The model under review builds one solid part; all positions refer to its coordinate system, in mm. Coordinates: 2 decimals unless noted, no trailing zeros. Write each loop counter-clockwise with the first axis right and the second up, starting at its lowest first coordinate (ties: lowest second). Pieces come first, ordered by that corner, then holes. Notation, with made-up numbers: (-15, -20) -> (0, -20) arc R8 ccw to (0, -8) -> close; hole circle Ø2 at (84.5, 24.25). An arc over 180 degrees is marked (long way). Put each result on its own line as item: value. Start each with the question number.
from build123d import *

# Parameters (mm, degrees)
F1_DEPTH = 10


with BuildPart() as f1:
    # F0 (on Top) → F1 (new body)
    with BuildSketch(Plane.XY):
        with BuildLine():
            Line((3.8890872965, 3.8890872965), (3.1819805153, 3.1819805153))
            ThreePointArc((3.1819805153, 3.1819805153), (4.1574578963, 1.7220754456), (4.5, 0))
            ThreePointArc((4.5, 0), (3.1819805153, -3.1819805153), (0, -4.5))
            Line((0, -4.5), (0, -5.5))
            ThreePointArc((0, -5.5), (3.8890872965, -3.8890872965), (5.5, 0))
            ThreePointArc((5.5, 0), (5.0813374288, 2.104758878), (3.8890872965, 3.8890872965))
        make_face()
        with BuildLine():
            Line((4.5961940777, 4.5961940777), (3.8890872965, 3.8890872965))
            ThreePointArc((3.8890872965, 3.8890872965), (5.0813374288, 2.104758878), (5.5, 0))
            ThreePointArc((5.5, 0), (3.8890872965, -3.8890872965), (0, -5.5))
            Line((0, -5.5), (0, -6.5))
            ThreePointArc((0, -6.5), (4.5961940777, -4.5961940777), (6.5, 0))
            ThreePointArc((6.5, 0), (6.0052169613, 2.4874423104), (4.5961940777, 4.5961940777))
        make_face()
        with BuildLine():
            Line((5.6568542495, 5.6568542495), (4.5961940777, 4.5961940777))
            ThreePointArc((4.5961940777, 4.5961940777), (6.0052169613, 2.4874423104), (6.5, 0))
            ThreePointArc((6.5, 0), (4.5961940777, -4.5961940777), (0, -6.5))
            Line((0, -6.5), (0, -8))
            ThreePointArc((0, -8), (5.6568542495, -5.6568542495), (8, 0))
            ThreePointArc((8, 0), (7.3910362601, 3.0614674589), (5.6568542495, 5.6568542495))
        make_face()
        with BuildLine():
            Line((6.3639610307, 6.3639610307), (5.6568542495, 5.6568542495))
            ThreePointArc((5.6568542495, 5.6568542495), (7.3910362601, 3.0614674589), (8, 0))
            ThreePointArc((8, 0), (5.6568542495, -5.6568542495), (0, -8))
            Line((0, -8), (0, -9))
            ThreePointArc((0, -9), (6.3639610307, -6.3639610307), (9, 0))
            ThreePointArc((9, 0), (8.3149157926, 3.4441508913), (6.3639610307, 6.3639610307))
        make_face()
        with BuildLine():
            Line((8.8388347648, 8.8388347648), (7.4246212025, 7.4246212025))
            ThreePointArc((7.4246212025, 7.4246212025), (9.7007350914, 4.0181760398), (10.5, 0))
            ThreePointArc((10.5, 0), (7.4246212025, -7.4246212025), (0, -10.5))
            Line((0, -10.5), (0, -12.5))
            ThreePointArc((0, -12.5), (8.8388347648, -8.8388347648), (12.5, 0))
            ThreePointArc((12.5, 0), (11.5484941564, 4.7835429046), (8.8388347648, 8.8388347648))
        make_face()
        with BuildLine():
            ThreePointArc((-10.5, 0), (-4.0181760398, 9.7007350914), (7.4246212025, 7.4246212025))
            Line((7.4246212025, 7.4246212025), (8.8388347648, 8.8388347648))
            ThreePointArc((8.8388347648, 8.8388347648), (-4.7835429046, 11.5484941564), (-12.5, 0))
            Line((-12.5, 0), (-10.5, 0))
        make_face()
        with BuildLine():
            ThreePointArc((-9, 0), (-3.4441508913, 8.3149157926), (6.3639610307, 6.3639610307))
            Line((6.3639610307, 6.3639610307), (7.4246212025, 7.4246212025))
            ThreePointArc((7.4246212025, 7.4246212025), (-4.0181760398, 9.7007350914), (-10.5, 0))
            Line((-10.5, 0), (-9, 0))
        make_face()
        with BuildLine():
            ThreePointArc((-8, 0), (-3.0614674589, 7.3910362601), (5.6568542495, 5.6568542495))
            Line((5.6568542495, 5.6568542495), (6.3639610307, 6.3639610307))
            ThreePointArc((6.3639610307, 6.3639610307), (-3.4441508913, 8.3149157926), (-9, 0))
            Line((-9, 0), (-8, 0))
        make_face()
        with BuildLine():
            ThreePointArc((-6.5, 0), (-2.4874423104, 6.0052169613), (4.5961940777, 4.5961940777))
            Line((4.5961940777, 4.5961940777), (5.6568542495, 5.6568542495))
            ThreePointArc((5.6568542495, 5.6568542495), (-3.0614674589, 7.3910362601), (-8, 0))
            Line((-8, 0), (-6.5, 0))
        make_face()
        with BuildLine():
            Line((7.4246212025, 7.4246212025), (6.3639610307, 6.3639610307))
            ThreePointArc((6.3639610307, 6.3639610307), (8.3149157926, 3.4441508913), (9, 0))
            ThreePointArc((9, 0), (6.3639610307, -6.3639610307), (0, -9))
            Line((0, -9), (0, -10.5))
            ThreePointArc((0, -10.5), (7.4246212025, -7.4246212025), (10.5, 0))
            ThreePointArc((10.5, 0), (9.7007350914, 4.0181760398), (7.4246212025, 7.4246212025))
        make_face()
        with BuildLine():
            ThreePointArc((-4.5, 0), (-1.7220754456, 4.1574578963), (3.1819805153, 3.1819805153))
            Line((3.1819805153, 3.1819805153), (3.8890872965, 3.8890872965))
            ThreePointArc((3.8890872965, 3.8890872965), (-2.104758878, 5.0813374288), (-5.5, 0))
            Line((-5.5, 0), (-4.5, 0))
        make_face()
        with BuildLine():
            ThreePointArc((-5.5, 0), (-2.104758878, 5.0813374288), (3.8890872965, 3.8890872965))
            Line((3.8890872965, 3.8890872965), (4.5961940777, 4.5961940777))
            ThreePointArc((4.5961940777, 4.5961940777), (-2.4874423104, 6.0052169613), (-6.5, 0))
            Line((-6.5, 0), (-5.5, 0))
        make_face()
        with BuildLine():
            ThreePointArc((2.8284271247, 2.8284271247), (3.69551813, 1.5307337295), (4, 0))
            ThreePointArc((4, 0), (2.8284271247, -2.8284271247), (0, -4))
            Line((0, -4), (0, -4.5))
            ThreePointArc((0, -4.5), (3.1819805153, -3.1819805153), (4.5, 0))
            ThreePointArc((4.5, 0), (4.1574578963, 1.7220754456), (3.1819805153, 3.1819805153))
            Line((3.1819805153, 3.1819805153), (2.8284271247, 2.8284271247))
        make_face()
        with BuildLine():
            ThreePointArc((-4, 0), (-1.5307337295, 3.69551813), (2.8284271247, 2.8284271247))
            Line((2.8284271247, 2.8284271247), (3.1819805153, 3.1819805153))
            ThreePointArc((3.1819805153, 3.1819805153), (-1.7220754456, 4.1574578963), (-4.5, 0))
            Line((-4.5, 0), (-4, 0))
        make_face()
        with BuildLine():
            Line((0, -4.5), (0, -4))
            ThreePointArc((0, -4), (-2.8284271247, -2.8284271247), (-4, 0))
            Line((-4, 0), (-4.5, 0))
            ThreePointArc((-4.5, 0), (-3.1819805153, -3.1819805153), (0, -4.5))
        make_face()
        with BuildLine():
            Line((0, -5.5), (0, -4.5))
            ThreePointArc((0, -4.5), (-3.1819805153, -3.1819805153), (-4.5, 0))
            Line((-4.5, 0), (-5.5, 0))
            ThreePointArc((-5.5, 0), (-3.8890872965, -3.8890872965), (0, -5.5))
        make_face()
        with BuildLine():
            Line((0, -6.5), (0, -5.5))
            ThreePointArc((0, -5.5), (-3.8890872965, -3.8890872965), (-5.5, 0))
            Line((-5.5, 0), (-6.5, 0))
            ThreePointArc((-6.5, 0), (-4.5961940777, -4.5961940777), (0, -6.5))
        make_face()
        with BuildLine():
            Line((0, -8), (0, -6.5))
            ThreePointArc((0, -6.5), (-4.5961940777, -4.5961940777), (-6.5, 0))
            Line((-6.5, 0), (-8, 0))
            ThreePointArc((-8, 0), (-5.6568542495, -5.6568542495), (0, -8))
        make_face()
        with BuildLine():
            Line((0, -9), (0, -8))
            ThreePointArc((0, -8), (-5.6568542495, -5.6568542495), (-8, 0))
            Line((-8, 0), (-9, 0))
            ThreePointArc((-9, 0), (-6.3639610307, -6.3639610307), (0, -9))
        make_face()
        with BuildLine():
            Line((0, -10.5), (0, -9))
            ThreePointArc((0, -9), (-6.3639610307, -6.3639610307), (-9, 0))
            Line((-9, 0), (-10.5, 0))
            ThreePointArc((-10.5, 0), (-7.4246212025, -7.4246212025), (0, -10.5))
        make_face()
        with BuildLine():
            Line((0, -12.5), (0, -10.5))
            ThreePointArc((0, -10.5), (-7.4246212025, -7.4246212025), (-10.5, 0))
            Line((-10.5, 0), (-12.5, 0))
            ThreePointArc((-12.5, 0), (-8.8388347648, -8.8388347648), (0, -12.5))
        make_face()
    extrude(amount=-F1_DEPTH)


solid = f1.part
1. Consider section A-A on z = -6.5. State the section outline as (x, y) points, then the cut area to 3 significant figures.
2. Consider section C-C on y = -10. State the section outline as (x, z) points.
3. Insertion check: P1, Ø3, axis at y = 1.5, z = -6, coming from the +X side; P2, Ø2, axis at y = -4.5, z = -7.5, coming from the -X side; P3, Ø3, axis at y = 4.5, z = -7.5, coming from the +X side. Each pin has a flat end and moves straight along its axis. Give the tip position at first contact, or say it passes through.
4. Consider section B-B on y = -1. State the section outline as (x, z) points.
5. Wall thickness on line 1 (Y direction, x = 0.25, z = -0.5); line 2 (X direction, y = -1.75, z = -7.75): over which ranges is each line inside the solid? List them lowest first. Write a range as from..to.
6. Consider section D-D on x = -9.5. State the section outline as (y, z) points.
Output values:
1. outline: circle Ø25 at (0, 0); hole circle Ø8 at (0, 0)
1. area: 441 mm^2
2. outline: (-7.5, -10) -> (7.5, -10) -> (7.5, 0) -> (-7.5, 0) -> close
3. P1: stops at x = 12.5
3. P2: stops at x = -12
3. P3: stops at x = 12.13
4. outline: (-12.46, -10) -> (-3.87, -10) -> (-3.87, 0) -> (-12.46, 0) -> close; (3.87, -10) -> (12.46, -10) -> (12.46, 0) -> (3.87, 0) -> close
5. line 1: y = -12.5..-3.99, 3.99..12.5
5. line 2: x = -12.38..-3.6, 3.6..12.38
6. outline: (-8.12, -10) -> (8.12, -10) -> (8.12, 0) -> (-8.12, 0) -> close
